```python
from build123d import *

# Parameters (mm, degrees)
F0_R     = 1
F1_DEPTH = 6
F2_DEPTH = 9
F3_R     = 4


with BuildPart() as f1:
    # F0 (on Front) → F1 (new body, symmetric)
    with BuildSketch(Plane.XZ):
        with BuildLine():
            Line((0, 37.671893), (0, 25.4))
            ThreePointArc((0, 25.4), (5.298719, 24.841167), (10.364281, 23.189258))
            Line((10.364281, 23.189258), (10.364281, 25.364181))
            Line((10.364281, 25.364181), (10.364281, 33.899603))
            Line((10.364281, 33.899603), (7.517861, 34.935616))
            Line((7.517861, 34.935616), (0, 37.671893))
        make_face()
        with BuildLine():
            Line((2, 27.32691), (2, 34.815597))
            Line((2, 34.815597), (8.364471, 32.499119))
            Line((8.364471, 32.499119), (8.364471, 26.092061))
            ThreePointArc((8.364471, 26.092061), (5.218886, 26.898387), (2, 27.32691))
        make_face(mode=Mode.SUBTRACT)
        with BuildLine():
            Line((0, 40.284664), (0, 37.671893))
            Line((0, 37.671893), (7.517861, 34.935616))
            Line((7.517861, 34.935616), (7.517861, 40.284664))
            ThreePointArc((7.517861, 40.284664), (3.75893, 44.043594), (0, 40.284664))
        make_face()
        with Locations((3.75893, 40.284664)):
            Circle(F0_R, mode=Mode.SUBTRACT)
    extrude(amount=F1_DEPTH, both=True)

    # F0 (on Front) → F2 (join, symmetric)
    with BuildSketch(Plane.XZ):
        with BuildLine():
            Line((8.364471, 32.499119), (2, 34.815597))
            Line((2, 34.815597), (2, 27.32691))
            ThreePointArc((2, 27.32691), (5.218886, 26.898387), (8.364471, 26.092061))
            Line((8.364471, 26.092061), (8.364471, 32.499119))
        make_face()
    extrude(amount=F2_DEPTH, both=True)

    # F3
    f3_edges = [f1.edges().sort_by_distance(p)[0] for p in [
        (7.517861, 0, 34.935616),
    ]]
    fillet(f3_edges, radius=F3_R)


solid = f1.part
```
The listing builds one solid part. Answer for the finished solid, in the listing's coordinates (mm). A direction names the side the tool comes from. Coordinates: 2 decimals unless noted, no trailing zeros. Order: outer loops, then holes, each group sorted by start corner. A loop starts at its lowest first (then second) coordinate and runs counter-clockwise, first axis right, second up. Notation, with made-up numbers: M 8,79.25 L 20,79.25 A19 cw 20,103.25 Z; hole C -40,-10.75 d5. An arc over 180 degrees is marked long. Answer as a JSON object with one key per item and string values. Group by question number.
1. Straight lines are drawn through the part: line 1 (Y direction, x = 3.75, z = 27); line 2 (Z direction, x = 4.5, y = -1.25); line 3 (Z direction, x = 3, y = -3). For each, find the intervals that lie inside material, in ascending order.
2. Section A-A on y = 3.25 is taken. Write down the section's boundary in (x, z), then the cut area to 3 significant figures.
3. Section D-D on y = -6.5 is taken. Write down the section's boundary in (x, z), then the cut area to 3 significant figures.
4. Flat-ended cylindrical pins translate along their axes: P1, Ø2.5, axis at y = 7.5, z = 31, coming from the -X side; P2, Ø4, axis at x = 5.5, y = 1, coming from the +Z side; P3, Ø1, axis at x = 2.5, z = 26, coming from the -Y side; P4, Ø3, axis at y = -1, z = 39, coming from the +X side. Find the tip coordinate at first contact, or state that the pin passes through.
5. Section C-C on z = 30.5 is taken. Write down the section's boundary in (x, y), then the cut area to 3 significant figures.
6. Section B-B on x = 4.5 is taken. Write down the section's boundary in (y, z), then the cut area to 3 significant figures.
7. Determine the mould class of faces 1 (the cylindrical face through (3.54, 0.08, 39.31)), 2 (the cylindrical face through (5.174, 7.479, 26.907)), 3 (the flat face through (5, -6, 34)) for opening direction Z: released by +Z, released by -Z, zero draft, split by the parting line, or undercut.
8. A tool of negligible diameter and unlimited length cuts with its end or side. For faces 4 (the flat face through (5.23, 7.48, 33.64)), 5 (the flat face through (8.364, -8, 29)), 6 (the flat face through (2, -8, 31)), 7 (the flat face through (8.364, 7, 29)), from which of +Z, -Z, +X, -X, +Y, -Y can it reach the whole face along a straight path? Write none if from no direction.
Values follow:
{
 "1": {"line 1": "-6 to 6", "line 2": "25 to 39.61, 40.96 to 43.97", "line 3": "25.22 to 39.63, 40.94 to 43.97"},
 "2": {"outline": "M 0,25.4 A25.4 cw 10.36,23.19 L 10.36,33.9 L 10.15,33.98 A4 cw 7.52,37.74 L 7.52,40.28 A3.76 ccw 0,40.28 Z; hole C 3.76,40.28 d2", "area": "166 mm2"},
 "3": {"outline": "M 2,27.33 A27.4 cw 8.36,26.09 L 8.36,32.5 L 2,34.82 Z", "area": "43.4 mm2"},
 "4": {"P1": "x = 2", "P2": "z = 44.04", "P3": "y = -6", "P4": "x = 7.52"},
 "5": {"outline": "M 0,-6 L 2,-6 L 2,-9 L 8.36,-9 L 8.36,-6 L 10.36,-6 L 10.36,6 L 8.36,6 L 8.36,9 L 2,9 L 2,6 L 0,6 Z", "area": "163 mm2"},
 "6": {"outline": "M -9,27.03 L -6,27.03 L -6,25 L 6,25 L 6,27.03 L 9,27.03 L 9,33.91 L 6,33.91 L 6,39.61 L -6,39.61 L -6,33.91 L -9,33.91 Z; M -6,40.96 L 6,40.96 L 6,43.97 L -6,43.97 Z", "area": "253 mm2"},
 "7": {"face 1": "undercut", "face 2": "released by -Z", "face 3": "zero draft"},
 "8": {"face 4": "+Z, +X, +Y", "face 5": "+Z, -Z, +X, -Y", "face 6": "+Z, -Z, -X, -Y", "face 7": "+Z, -Z, +X, +Y"}
}
